For this review, take the finished solid that the model builds, in its own axes (mm). Face numbers are marked on the shaded views. A direction names the side the tool comes from. Coordinates: 2 decimals unless noted, no trailing zeros. Loops run counter-clockwise (first coordinate to the right, second up) from the corner with the lowest first, then second, coordinate; pieces in that order, holes last. Notation, with made-up numbers: (49, 8) -> (93, 8) arc R30 cw to (93, 30) -> close; hole circle Ø2 at (-11, 85). An arc over 180 degrees is marked (long way). Use a Markdown table: item, result.
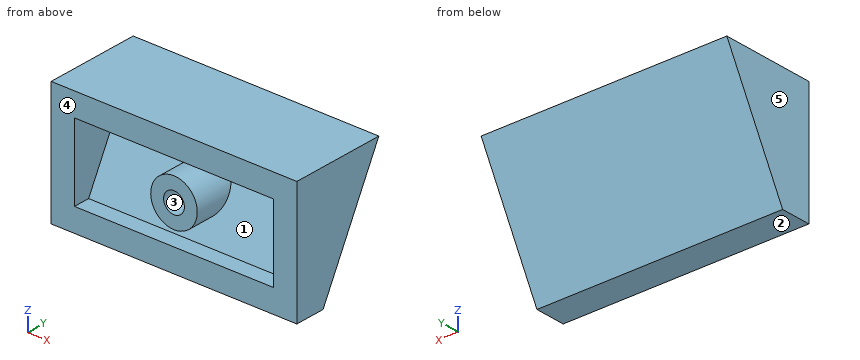
from build123d import *

# Parameters (mm, degrees)
BOSS_EXTRUDE1_DEPTH = 15.83
SHELL1_T            = -1.5
BOSS_EXTRUDE3_REACH = 20.742
SKETCH2_R           = 1.5
SKETCH2_R_2         = 0.67


with BuildPart() as part:
    # Sketch1 → Boss-Extrude1 (new body)
    with BuildSketch(Plane(origin=(0, 0, 0), x_dir=(0, 0, -1), z_dir=(1, 0, 0))):
        Polygon((0, 0), (0, 6.16), (7.92, 1.97), (7.92, 0), align=None)
    extrude(amount=BOSS_EXTRUDE1_DEPTH)

    # Shell1
    shell1_openings = [part.faces().sort_by_distance(p)[0] for p in [
        (7.915, 0, -3.96),
    ]]
    offset(amount=SHELL1_T, openings=shell1_openings, kind=Kind.INTERSECTION)

    # Boss-Extrude3: up to this plane
    boss_extrude3_end = Plane(origin=(15.83, 0.644114575, -7.218553039), z_dir=(0, -0.8839236168124106, 0.46763130737929287))
    # Sketch2 → Boss-Extrude3 (add, up to the surface)
    with BuildSketch(Plane(origin=(0, 0, 0), x_dir=(1, 0, 0), z_dir=(0, 1, 0)), mode=Mode.PRIVATE) as boss_extrude3_sk1:
        with Locations(Location((7.915, 3.96, 0), (0, 0, 90))):
            Circle(SKETCH2_R)
        with Locations(Location((7.915, 3.96, 0), (0, 0, 90))):
            Circle(SKETCH2_R_2, mode=Mode.SUBTRACT)
    boss_extrude3_tool1 = split(extrude(boss_extrude3_sk1.sketch, amount=BOSS_EXTRUDE3_REACH, mode=Mode.PRIVATE), bisect_by=boss_extrude3_end, keep=Keep.BOTH, mode=Mode.PRIVATE)
    add(boss_extrude3_tool1.solids().sort_by_distance((7.915, 0, -2.502426))[0])


solid = part.part
(1) For the marked faces 1 and 2, list the 3-axis set-ups (+Z, -Z, +X, -X, +Y, -Y) from which the entire face can be reached by the end or side of a thin tool; tool diameter is ignored.
Found:
| item | result |
|---|---|
| face 1 | -Y |
| face 2 | -Z, +X, -X, +Y, -Y |
(2) Mouldability with a two-part tool opening along X and no side actions: class the marked faces 3, 4 and 5 as pulls with the +X half, pulls with the -X half, needs draft (parallel to the pull), parting line crosses it, or undercut.
Found:
| item | result |
|---|---|
| face 3 | undercut |
| face 4 | needs draft |
| face 5 | pulls with the -X half |
(3) Take a section at D-D on x = 7.75. Write out the cut boundary in (y, z), plus the area to 3 significant figures.
Found:
| item | result |
|---|---|
| outline | (0, -7.92) -> (1.97, -7.92) -> (6.16, 0) -> (0, 0) -> (0, -1.5) -> (3.67, -1.5) -> (3.16, -2.47) -> (0, -2.47) -> (0, -3.31) -> (2.71, -3.31) -> (2.02, -4.61) -> (0, -4.61) -> (0, -5.45) -> (1.58, -5.45) -> (1.07, -6.42) -> (0, -6.42) -> close |
| area | 24.5 mm^2 |
(4) Take a section at B-B on z = -2. Write out the cut boundary in (x, y), plus the area to 3 significant figures.
Found:
| item | result |
|---|---|
| outline | (0, 0) -> (1.5, 0) -> (1.5, 3.4) -> (14.33, 3.4) -> (14.33, 0) -> (15.83, 0) -> (15.83, 5.1) -> (0, 5.1) -> close |
| area | 37.1 mm^2 |
(5) For pin 1 Ø1.5 at (x, z) = (11.5, -4.5) entering from -Y, flat-tipped, find the tip position at first contact; note if it passes through.
Found:
| item | result |
|---|---|
| pin 1 | stops at y = 1.69 |
(6) Take a section at A-A on x = 4.75. Write out the cut boundary in (y, z), plus the area to 3 significant figures.
Found:
| item | result |
|---|---|
| outline | (0, -7.92) -> (1.97, -7.92) -> (6.16, 0) -> (0, 0) -> (0, -1.5) -> (3.67, -1.5) -> (1.07, -6.42) -> (0, -6.42) -> close |
| area | 20.5 mm^2 |
(7) Take a section at C-C on z = -3.96. Write out the cut boundary in (x, y) (3 decimals), plus the area to 3 significant figures.
Found:
| item | result |
|---|---|
| outline | (0, 0) -> (1.5, 0) -> (1.5, 2.368) -> (6.415, 2.368) -> (6.415, 0) -> (7.245, 0) -> (7.245, 2.368) -> (8.585, 2.368) -> (8.585, 0) -> (9.415, 0) -> (9.415, 2.368) -> (14.33, 2.368) -> (14.33, 0) -> (15.83, 0) -> (15.83, 4.065) -> (0, 4.065) -> close |
| area | 37.9 mm^2 |
(8) For line 1 along X through (y, z) = (1.35, -3.96) (3 decimals); line 2 along Z through (x, y) = (4.5, 0.75); line 3 along Z through (x, y) = (8.25, 1.25), list the stretches that pass through material, from the lowest coordinate up.
Found:
| item | result |
|---|---|
| line 1 | x = 0 to 1.5, 6.415 to 7.245, 8.585 to 9.415, 14.33 to 15.83 |
| line 2 | z = -7.92 to -6.42, -1.5 to 0 |
| line 3 | z = -7.92 to -6.07, -5.42 to -4.54, -3.38 to -2.5, -1.5 to 0 |
